Part model, mm, in its own coordinate system. Face numbers are marked on the shaded views. A direction names the side the tool comes from. Round coordinates to 2 decimals unless told otherwise and drop trailing zeros. Write each loop counter-clockwise with the first axis right and the second up, starting at its lowest first coordinate (ties: lowest second). Pieces come first, ordered by that corner, then holes. Notation, with made-up numbers: M 35.5,73 L 76.5,73 A21 ccw 76.5,105 Z; hole C 88.5,-31.5 d11. An arc over 180 degrees is marked long. Use a Markdown table: item, result. Add a question column.
1) Slice it at D-D on y = 17. Write the cut outline in (x, z), plus the area to 3 significant figures.
2) Two-plate mould, pull along X, no slides. Class the marked faces 1, 2 and 3: released by +X, released by -X, zero draft, split by the parting line, or undercut.
3) Which spindle directions (+Z, -Z, +X, -X, +Y, -Y) get a long thin tool onto all of the face, cutting with end or side? Do the marked faces 4, 5, 6, 7 and 8. Say none if no direction does.
4) Drop flat-ended pins along their axis: P1, Ø2, axis at y = 14.5, z = -1.5, coming from the -X side; P2, Ø6, axis at y = 28.5, z = 6, coming from the -X side; P3, Ø4, axis at x = -8, y = 10.5, coming from the -Z side; P4, Ø8, axis at x = -9.5, y = 19.5, coming from the +Z side. Give the stop position or say it passes through.
5) Slice it at A-A on y = 21. Write the cut outline in (x, z) (3 decimals), plus the area to 3 significant figures.
6) Slice it at B-B on z = 6.35. Write the cut outline in (x, y) (3 decimals), plus the area to 3 significant figures.
7) Slice it at C-C on x = -6.35. Write the cut outline in (y, z) (3 decimals), plus the area to 3 significant figures.
8) Wall check: probe 1 along Z at (x, y) = (-12.5, 26); probe 2 along Y at (x, z) = (-2.45, 6.35); probe 3 along X at (y, z) = (26.5, 9.5). Give the ranges that are in metal, low to high.
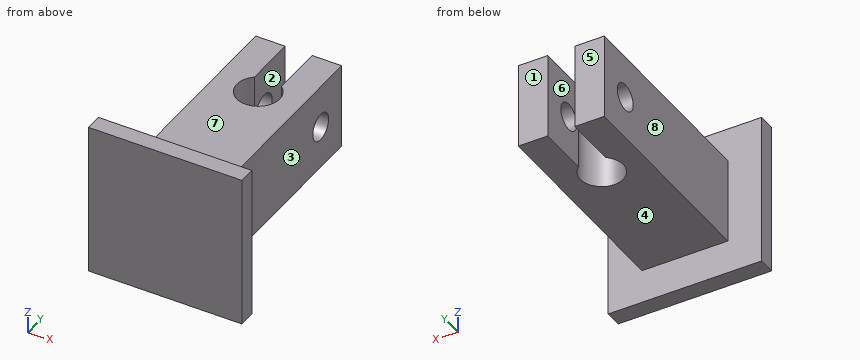
```python
from build123d import *

# Parameters (mm, degrees)
BOSS_EXTRUDE1_DEPTH = 12.7
SKETCH2_W           = 22.7
SKETCH2_H           = 22.7
BOSS_EXTRUDE2_DEPTH = 2.5
SKETCH3_R           = 2
CUT_EXTRUDE1_DEPTH  = 18.7


with BuildPart() as part:
    # Sketch1 → Boss-Extrude1 (new body)
    with BuildSketch(Plane.XY):
        with BuildLine():
            Line((0, 0), (0, 31.2))
            Line((0, 31.2), (-4.35, 31.2))
            Line((-4.35, 31.2), (-4.35, 23.465892333))
            ThreePointArc((-4.35, 23.465892333), (-6.35, 17.825), (-8.35, 23.465892333))
            Line((-8.35, 23.465892333), (-8.35, 31.2))
            Line((-8.35, 31.2), (-12.7, 31.2))
            Line((-12.7, 31.2), (-12.7, 0))
            Line((-12.7, 0), (0, 0))
        make_face()
    extrude(amount=BOSS_EXTRUDE1_DEPTH)

    # Sketch2 → Boss-Extrude2 (add)
    with BuildSketch(Plane.XZ):
        with Locations((-6.35, 6.35)):
            Rectangle(SKETCH2_W, SKETCH2_H)
    extrude(amount=BOSS_EXTRUDE2_DEPTH)

    # Sketch3 → Cut-Extrude1 (cut, through all)
    with BuildSketch(Plane(origin=(0, 0, 0), x_dir=(0, 0, -1), z_dir=(1, 0, 0))):
        with Locations((-6.35, 25.920446167)):
            Circle(SKETCH3_R)
    extrude(amount=-CUT_EXTRUDE1_DEPTH, mode=Mode.SUBTRACT)


solid = part.part
```
Entries:
| question | item | result |
|---|---|---|
| 1 | outline | M -12.7,0 L 0,0 L 0,12.7 L -12.7,12.7 Z |
| 1 | area | 161 mm^2 |
| 2 | face 1 | zero draft |
| 2 | face 2 | undercut |
| 2 | face 3 | released by +X |
| 3 | face 4 | -Z, +X, -X, +Y |
| 3 | face 5 | +Z, -Z, +X, -X, +Y |
| 3 | face 6 | +Z, -Z, +Y |
| 3 | face 7 | +Z, +X, -X, +Y |
| 3 | face 8 | +Z, -Z, -X, +Y |
| 4 | P1 | passes through |
| 4 | P2 | stops at x = -12.7 |
| 4 | P3 | stops at z = 0 |
| 4 | P4 | stops at z = 12.7 |
| 5 | outline | M -12.7,0 L -9.525,0 L -9.525,12.7 L -12.7,12.7 Z; M -3.175,0 L 0,0 L 0,12.7 L -3.175,12.7 Z |
| 5 | area | 80.6 mm^2 |
| 6 | outline | M -17.7,-2.5 L 5,-2.5 L 5,0 L 0,0 L 0,23.92 L -4.35,23.92 L -4.35,23.466 A3.175 cw long -8.35,23.466 L -8.35,23.92 L -12.7,23.92 L -12.7,0 L -17.7,0 Z; M -12.7,27.92 L -8.35,27.92 L -8.35,31.2 L -12.7,31.2 Z; M -4.35,27.92 L 0,27.92 L 0,31.2 L -4.35,31.2 Z |
| 6 | area | 358 mm^2 |
| 7 | outline | M -2.5,-5 L 0,-5 L 0,0 L 17.825,0 L 17.825,12.7 L 0,12.7 L 0,17.7 L -2.5,17.7 Z |
| 7 | area | 283 mm^2 |
| 8 | probe 1 | z = 0 to 4.35, 8.35 to 12.7 |
| 8 | probe 2 | y = -2.5 to 23.92, 27.92 to 31.2 |
| 8 | probe 3 | x = -12.7 to -8.35, -4.35 to 0 |
